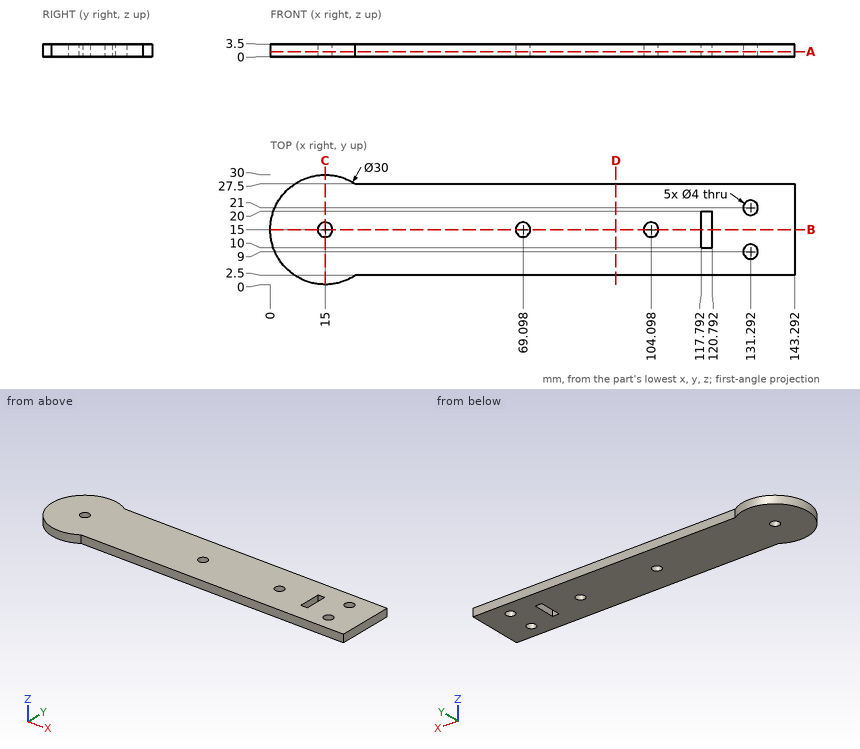
For this review, use the dimensioned drawing (mm, ordinates from the lowest corner) and the shaded views. Coordinates: 2 decimals unless noted, no trailing zeros. Order: outer loops, then holes, each group sorted by start corner. A loop starts at its lowest first (then second) coordinate and runs counter-clockwise, first axis right, second up. Notation, with made-up numbers: (-31.5, 8) -> (25.5, 8) arc R29 cw to (25.5, 43) -> close; hole circle Ø10 at (52, 10). An arc over 180 degrees is marked (long way). One line per item, written item: value. Start each with the question number.
Q1. Take a section at D-D, the plane x = 94.5. State the section outline as (y, z) points.
Q2. Take a section at C-C, the plane x = 15. State the section outline as (y, z) points.
Q3. Take a section at A-A, the plane z = 1.45. State the section outline as (x, y) points, then the cut area to 3 significant figures.
Q4. Insertion check: pin 1 Ø1.5 at (x, z) = (119, 2) entering from -Y; pin 2 Ø0.9 at (x, z) = (120, 2) entering from +Y. Each pin has a flat end and moves straight along its axis. Give the tip position at first contact, or say it passes through.
Q5. For probe 1 along X at (y, z) = (15, 2.2); probe 2 along X at (y, z) = (14, 0.45) (1 decimal); probe 3 along Y at (x, z) = (15, 1.2), list the stretches that pass through material, from the lowest coordinate up.
Q6. Take a section at B-B, the plane y = 15. State the section outline as (x, z) points, then the cut area to 3 significant figures.
Values follow:
1. outline: (2.5, 0) -> (27.5, 0) -> (27.5, 3.5) -> (2.5, 3.5) -> close
2. outline: (0, 0) -> (13, 0) -> (13, 3.5) -> (0, 3.5) -> close; (17, 0) -> (30, 0) -> (30, 3.5) -> (17, 3.5) -> close
3. outline: (23.29, 2.5) -> (143.29, 2.5) -> (143.29, 27.5) -> (23.29, 27.5) arc R15 ccw (long way) to start; hole circle Ø4 at (15, 15); hole circle Ø4 at (69.1, 15); hole circle Ø4 at (104.1, 15); hole (117.79, 10) -> (120.79, 10) -> (120.79, 20) -> (117.79, 20) -> close; hole circle Ø4 at (131.29, 9); hole circle Ø4 at (131.29, 21)
3. area: 3,500 mm2
4. pin 1: stops at y = 2.5
4. pin 2: stops at y = 27.5
5. probe 1: x = 0 to 13, 17 to 67.1, 71.1 to 102.1, 106.1 to 117.79, 120.79 to 143.29
5. probe 2: x = 0 to 13.3, 16.7 to 67.4, 70.8 to 102.4, 105.8 to 117.8, 120.8 to 143.3
5. probe 3: y = 0 to 13, 17 to 30
6. outline: (0, 0) -> (13, 0) -> (13, 3.5) -> (0, 3.5) -> close; (17, 0) -> (67.1, 0) -> (67.1, 3.5) -> (17, 3.5) -> close; (71.1, 0) -> (102.1, 0) -> (102.1, 3.5) -> (71.1, 3.5) -> close; (106.1, 0) -> (117.79, 0) -> (117.79, 3.5) -> (106.1, 3.5) -> close; (120.79, 0) -> (143.29, 0) -> (143.29, 3.5) -> (120.79, 3.5) -> close
6. area: 449 mm2
